from build123d import *

# Parameters (mm, degrees)
SKETCH_1_R        = 8
SKETCH_1_R_2      = 3.1
EXTRUDE_1_DEPTH   = 5
SKETCH_1_W        = 40
SKETCH_1_H        = 5
EXTRUDE_1_2_DEPTH = 5
CHAMFER_7_SIZE    = 0.5
EXTRUDE1_START    = -10
EXTRUDE1_DEPTH    = 10
FILLET1_R         = 3
EXTRUDE2_START    = -4.5
EXTRUDE2_DEPTH    = 4.5
FILLET2_R         = 8
SKETCH3_R         = 2.1
EXTRUDE3_DEPTH    = 29.869431931
CHAMFER2_SIZE     = 0.2
EXTRUDE4_DEPTH    = 27.952441448
FILLET3_R         = 2.5
FILLET4_R         = 3
CHAMFER4_SIZE     = 0.5


with BuildPart() as part:
    # 草图1 → 凸台-拉伸1 (new, symmetric)
    with BuildSketch(Plane.XY):
        Circle(SKETCH_1_R)
        Circle(SKETCH_1_R_2, mode=Mode.SUBTRACT)
    extrude(amount=EXTRUDE_1_DEPTH, both=True)

    # 倒角7
    chamfer_7_edges = [part.edges().sort_by_distance(p)[0] for p in [
        (-3.1, 0, -5),
        (-3.1, 0, 5),
    ]]
    chamfer(chamfer_7_edges, length=CHAMFER_7_SIZE)



with BuildPart() as body_2:
    # 草图1 → Extrude 1 2 (new, symmetric)
    with BuildSketch(Plane.XY):
        with Locations((0, -14.71)):
            Rectangle(SKETCH_1_W, SKETCH_1_H)
    extrude(amount=EXTRUDE_1_2_DEPTH, both=True)


with BuildPart() as part_1:
    add(part.part)

    add(body_2.part)  # Extrude1 merges body 2
    # Sketch1 → Extrude1 (add)
    with BuildSketch(Plane(origin=(0, 0, -5), x_dir=(-1, 0, 0), z_dir=(0, 0, -1)).offset(EXTRUDE1_START)):
        with BuildLine():
            ThreePointArc((8, 0), (0, -8), (-8, 0))
            Line((-8, 0), (-8, -12.21))
            Line((-8, -12.21), (8, -12.21))
            Line((8, -12.21), (8, 0))
        make_face()
    extrude(amount=EXTRUDE1_DEPTH)

    # Fillet1
    fillet1_edges = [part_1.edges().sort_by_distance(p)[0] for p in [
        (8, -12.21, 0),
        (-8, -12.21, 0),
    ]]
    fillet(fillet1_edges, radius=FILLET1_R)

    # Sketch2 → Extrude2 (cut)
    with BuildSketch(Plane(origin=(0, 0, -5), x_dir=(-1, 0, 0), z_dir=(0, 0, -1)).offset(EXTRUDE2_START)):
        with BuildLine():
            ThreePointArc((3, -7.416198487), (0, -8), (-3, -7.416198487))
            Line((-3, -7.416198487), (-3, -17.21))
            Line((-3, -17.21), (3, -17.21))
            Line((3, -17.21), (3, -7.416198487))
        make_face()
    extrude2 = extrude(amount=EXTRUDE2_DEPTH, mode=Mode.SUBTRACT)

    # Mirror1: Extrude2 across plane
    add(extrude2.mirror(Plane.XY), mode=Mode.SUBTRACT)

    # Fillet2
    fillet2_edges = [part_1.edges().sort_by_distance(p)[0] for p in [
        (-3, -17.21, -2.75),
        (3, -17.21, -2.75),
        (3, -17.21, 2.75),
        (-3, -17.21, 2.75),
    ]]
    fillet(fillet2_edges, radius=FILLET2_R)

    # Sketch3 → Extrude3 (cut, through all)
    with BuildSketch(Plane(origin=(0, -12.21, 0), x_dir=(1, 0, 0), z_dir=(0, 1, 0))):
        with Locations(Location((15, 0, 0), (0, 0, 270))):
            Circle(SKETCH3_R)
        with Locations(Location((-15, 0, 0), (0, 0, 90))):
            Circle(SKETCH3_R)
    extrude(amount=-EXTRUDE3_DEPTH, mode=Mode.SUBTRACT)

    # Chamfer2
    chamfer2_edges = [part_1.edges().sort_by_distance(p)[0] for p in [
        (15, -17.21, -2.1),
        (15, -12.21, -2.1),
        (-15, -17.21, 2.1),
        (-15, -12.21, 2.1),
    ]]
    chamfer(chamfer2_edges, length=CHAMFER2_SIZE)

    # Sketch4 → Extrude4 (cut, through all)
    with BuildSketch(Plane(origin=(0, 0, -0.5), x_dir=(-1, 0, 0), z_dir=(0, 0, -1))):
        with BuildLine():
            Line((-11, -17.21), (11, -17.21))
            ThreePointArc((11, -17.21), (5.343145751, -14.866854249), (3, -9.21))
            Line((3, -9.21), (3, -7.416198487))
            ThreePointArc((3, -7.416198487), (0, -8), (-3, -7.416198487))
            Line((-3, -7.416198487), (-3, -9.21))
            ThreePointArc((-3, -9.21), (-5.343145751, -14.866854249), (-11, -17.21))
        make_face()
    extrude(amount=-EXTRUDE4_DEPTH, mode=Mode.SUBTRACT)

    # Fillet3
    fillet3_edges = [part_1.edges().sort_by_distance(p)[0] for p in [
        (-3, -7.416198487, 0),
        (3, -7.416198487, 0),
    ]]
    fillet(fillet3_edges, radius=FILLET3_R)

    # Fillet4
    fillet4_edges = [part_1.edges().sort_by_distance(p)[0] for p in [
        (20, -14.71, -5),
        (-20, -14.71, 5),
        (20, -14.71, 5),
        (-20, -14.71, -5),
    ]]
    fillet(fillet4_edges, radius=FILLET4_R)

    # Chamfer4
    chamfer4_edges = [part_1.edges().sort_by_distance(p)[0] for p in [
        (0, 8, 5),
        (0, -8, -5),
        (8, -4.605, -5),
        (0, -8, 5),
        (-5.697451281, -15.200240152, -5),
        (5.697451281, -15.200240152, 5),
        (-2.182501473, -8.567267514, -5),
        (-2.182501473, -8.567267514, 5),
        (8, -4.605, 5),
        (2.182501473, -8.567267514, -5),
        (2.182501473, -8.567267514, 5),
        (-14, -17.21, -5),
        (-14, -12.21, -5),
        (-14, -12.21, 5),
        (-20, -12.21, 0),
        (-19.121320344, -12.21, 4.121320344),
        (-19.121320344, -12.21, -4.121320344),
        (-20, -17.21, 0),
        (-14, -17.21, 5),
        (-19.121320344, -17.21, 4.121320344),
        (-19.121320344, -17.21, -4.121320344),
        (20, -12.21, 0),
        (20, -17.21, 0),
        (19.121320344, -12.21, 4.121320344),
        (19.121320344, -12.21, -4.121320344),
        (19.121320344, -17.21, 4.121320344),
        (19.121320344, -17.21, -4.121320344),
        (0, 8, -5),
        (-8, -4.605, 5),
        (-8, -4.605, -5),
        (14, -12.21, 5),
        (14, -12.21, -5),
        (-8.878679656, -11.331320344, -5),
        (-8.878679656, -11.331320344, 5),
        (8.878679656, -11.331320344, -5),
        (8.878679656, -11.331320344, 5),
        (14, -17.21, -5),
        (14, -17.21, 5),
        (-5.697451281, -15.200240152, 5),
        (5.697451281, -15.200240152, -5),
    ]]
    chamfer(chamfer4_edges, length=CHAMFER4_SIZE)


solid = part_1.part
Verification items for the finished model (mm, model axes). A direction names the side the tool comes from. Give positions to 0.01 mm unless a question says otherwise; leave off trailing zeros. Write each loop counter-clockwise with the first axis right and the second up, starting at its lowest first coordinate (ties: lowest second). Pieces come first, ordered by that corner, then holes. Notation, with made-up numbers: M 12.5,40 L 58.5,40 A13 ccw 58.5,57 Z; hole C 71,-10.5 d3. An arc over 180 degrees is marked long. Write item = value, one per line.
(1) Sectioned sample at C-C (y = -4.75). Record the cut outline in (x, z).
Found:
outline = M -8,-4.5 L -7.5,-5 L 7.5,-5 L 8,-4.5 L 8,4.5 L 7.5,5 L -7.5,5 L -8,4.5 Z
(2) Go/stop test with flat-tipped pins: pin 1 Ø1 at (x, y) = (-3, -13.5) entering from +Z; pin 2 Ø4 at (y, z) = (4.5, -0.5) entering from +X; pin 3 Ø2.5 at (x, z) = (-13.5, 1.5) entering from +Y; pin 4 Ø4 at (x, z) = (-11, -2.5) entering from +Y. Record where each tip stops, or that it passes through.
Found:
pin_1 = through
pin_2 = 7.6
pin_3 = -12.21
pin_4 = -11.45
(3) Sectioned sample at A-A (x = 0). Record the cut outline in (y, z), then the cut area to 3 significant figures.
Found:
outline = M -8,-4.5 L -7.5,-5 L -3.6,-5 L -3.1,-4.5 L -3.1,4.5 L -3.6,5 L -7.5,5 L -8,4.5 Z; M 3.1,-4.5 L 3.6,-5 L 7.5,-5 L 8,-4.5 L 8,4.5 L 7.5,5 L 3.6,5 L 3.1,4.5 Z
area = 97.0 mm2
(4) Access from +Z, -Z, +X, -X, +Y, -Y to the whole of each face (thin tool, end or side, straight path). Record for faces 1 (the face through (0, -4, 5)), 2 (the face through (5.88, -14.88, -4.86)), 3 (the face through (5.99, -14.98, 4.86)), 4 (the face through (8, -5, 0)).
Found:
face_1 = +Z, +X, -X, +Y, -Y
face_2 = -Z, -Y
face_3 = +Z, -Y
face_4 = +Z, -Z, +X, +Y
(5) Material ranges on line 1 (X direction, y = -0.5, z = -3.5); line 2 (Z direction, x = -15, y = -13.7); line 3 (X direction, y = -12.5, z = -3.75), recorded low to high.
Found:
line_1 = -8 to -3.06, 3.06 to 8
line_2 = -5 to -2.1, 2.1 to 5
line_3 = -19.17 to -3.71, 3.71 to 19.17
(6) Draft check along X on faces 5 (the face through (8.86, -11.31, -0.06)), 6 (the face through (1.43, -2.75, -0.06)), 7 (the face through (-8, -5, 0)). Enter one of: released by +X, released by -X, zero draft, split by the parting line, or undercut.
Found:
face_5 = released by +X
face_6 = undercut
face_7 = released by -X
(7) Sectioned sample at B-B (z = 0). Give the number of separate pieces and of enclosed holes in the cut face, then the cut area to 3 significant figures.
Found:
separate_pieces = 3
enclosed_holes = 1
area = 346 mm2
